Design review of the part built by this model. Coordinates are the model's own, in mm. Give positions to 0.01 mm unless a question says otherwise; leave off trailing zeros. Loops run counter-clockwise (first coordinate to the right, second up) from the corner with the lowest first, then second, coordinate; pieces in that order, holes last. Notation, with made-up numbers: (75.25, 53) - (97.25, 53) arc R27 ccw to (97.25, 92) - close; hole circle Ø4 at (88.5, 13). An arc over 180 degrees is marked (long way). Write each question's results on one line, items separated by ' | '.
Autodesk Inventor part; units mm, degrees
ref_plane "Work Plane1" through (101.6, 0, 0) normal (1, 0, 0) x (0, 1, 0)
ref_plane "Work Plane2" through (0, -101.6, 0) normal (0, 1, 0) x (-1, 0, 0)
ref_plane "Work Plane3" through (-101.6, 0, 0) normal (1, 0, 0) x (0, 1, 0)
sketch "Sketch1" plane through (0, 0, 0) normal (0, 0, 1) x (1, 0, 0)
  circle A0 centre (0, 0) radius 12.7
  dimension "d0" = 25.4
extrude "Extrusion1" add sketch "Sketch1" along normal blind 25.4
ref_plane "Work Plane1" through (101.6, 0, 0) normal (1, 0, 0) x (0, 1, 0)
sketch "Sketch2" plane through (101.6, 0, 0) normal (1, 0, 0) x (0, 1, 0)
  arc A0 (-11.5079, 0) -> (12.6852, 24.1379) centre (-20.2903, 32.9957) ccw
  arc A1 (-12.7911, 0) -> (12.6852, 25.3834) centre (-25.5599, 38.2921) ccw
  line L0 (12.6852, 25.3834) -> (12.6852, 24.1379)
  line L1 (-12.7911, 0) -> (-11.5079, 0)
  point P0 (0, 0)
extrude "Extrusion2" add sketch "Sketch2" against normal blind 101.6
ref_plane "Work Plane2" through (0, -101.6, 0) normal (0, 1, 0) x (-1, 0, 0)
sketch "Sketch3" plane through (0, -101.6, 0) normal (0, 1, 0) x (-1, 0, 0)
  arc A0 (-12.7444, 23.4755) -> (10.8958, 0) centre (18.9573, 31.7588) ccw
  arc A1 (-12.7444, 25.3315) -> (12.6542, 0) centre (22.7301, 35.5012) ccw
  line L0 (-12.7444, 25.3315) -> (-12.7444, 23.4755)
  line L1 (12.6542, 0) -> (10.8958, 0)
  point P0 (0, 0)
  dimension "d7" = 32.766
extrude "Extrusion3" add sketch "Sketch3" along normal blind 101.6
ref_plane "Work Plane3" through (-101.6, 0, 0) normal (1, 0, 0) x (0, 1, 0)
sketch "Sketch4" plane through (-101.6, 0, 0) normal (1, 0, 0) x (0, 1, 0)
  arc A0 (-12.7444, 23.4755) -> (10.8958, 0) centre (18.9573, 31.7588) ccw
  arc A1 (-12.7444, 25.3315) -> (12.6542, 0) centre (22.7301, 35.5012) ccw
  line L0 (-12.7444, 25.3315) -> (-12.7444, 23.4755)
  line L1 (12.6542, 0) -> (10.8958, 0)
  point P0 (0, 0)
  point P1 (0, 0)
  dimension "d11" = 32.766
extrude "Extrusion4" add sketch "Sketch4" along normal blind 101.6
ref_plane "Work Plane4" through (0, 101.6, 0) normal (0, 1, 0) x (-1, 0, 0)
sketch "Sketch5" plane through (0, 101.6, 0) normal (0, 1, 0) x (-1, 0, 0)
  arc A0 (-11.5079, 0) -> (12.6852, 24.1379) centre (-20.2903, 32.9957) ccw
  arc A1 (-12.7911, 0) -> (12.6852, 25.3834) centre (-25.5599, 38.2921) ccw
  line L0 (12.6852, 25.3834) -> (12.6852, 24.1379)
  line L1 (-12.7911, 0) -> (-11.5079, 0)
  point P0 (0, 0)
  point P1 (0, 0)
extrude "Extrusion5" add sketch "Sketch5" against normal blind 101.6
properties part number "Fan"
(1) Draft analysis for pull direction Z (two halves, no side actions). For faces 1 (the flat face through (0, 0, 25.4)), 2 (the flat face through (-3, 101.6, 9)), state which applies: pulls with the +Z half, pulls with the -Z half, needs draft (parallel to the pull), parting line crosses it, or undercut.
Answers below:
face 1: pulls with the +Z half | face 2: needs draft
(2) Wall thickness on line 1 along Y through (x, z) = (-23, 14.25); line 2 along Y through (x, z) = (57, 23); line 3 along X through (y, z) = (-18.5, 19.25): over which ranges is each line inside the solid? List them lowest first. Write a range as from..to.
Answers below:
line 1: -8.74..-7.44 | line 2: 11.8..12.36 | line 3: 10.4..11.33
(3) Take a section at C-C on y = -59.5. Give the boundary of the cut face in (x, z).
Answers below:
outline: (-12.65, 0) - (-10.9, 0) arc R32.77 ccw to (12.74, 23.48) - (12.74, 25.33) arc R36.9 cw to start
(4) Take a section at A-A on z = 19.75. Give the boundary of the cut face in (x, y).
Answers below:
outline: (-101.6, -11.53) - (-5.33, -11.53) arc R12.7 ccw to (10.64, -6.93) - (10.64, -101.6) - (11.53, -101.6) - (11.53, -5.33) arc R12.7 ccw to (7.44, 10.29) - (101.6, 10.29) - (101.6, 11.18) - (6.02, 11.18) arc R12.7 ccw to (-10.29, 7.44) - (-10.29, 101.6) - (-11.18, 101.6) - (-11.18, 6.02) arc R12.7 ccw to (-6.93, -10.64) - (-101.6, -10.64) - close
(5) Take a section at B-B on x = -19. Give the boundary of the cut face in (y, z), plus the area to 3 significant figures.
Answers below:
outline: (-12.74, 23.48) arc R32.77 ccw to (10.9, 0) - (12.65, 0) arc R36.9 cw to (-12.74, 25.33) - close | area: 34.0 mm2
(6) Insertion check: P1, Ø0.6, axis at x = -29.5, z = 25, coming from the -Y side; P2, Ø8, axis at y = -80, z = 11.5, coming from the -X side; P3, Ø3, axis at y = 51.5, z = 9, coming from the -X side. Each pin has a flat end and moves straight along its axis. Give the tip position at first contact, or say it passes through.
Answers below:
P1: y = -12.74 | P2: x = 1.31 | P3: x = -5.4
